Can you work these out from the drawing? Everything is in mm from the part's minimum corner. A direction names the side the tool comes from. Coordinates: 2 decimals unless noted, no trailing zeros. Order: outer loops, then holes, each group sorted by start corner. A loop starts at its lowest first (then second) coordinate and runs counter-clockwise, first axis right, second up. Notation, with made-up numbers: (-16.75, 70) -> (12.25, 70) arc R29 ccw to (12.25, 90) -> close; hole circle Ø5 at (-8.75, 30). An arc over 180 degrees is marked (long way). Answer in a Markdown table with one row per item.
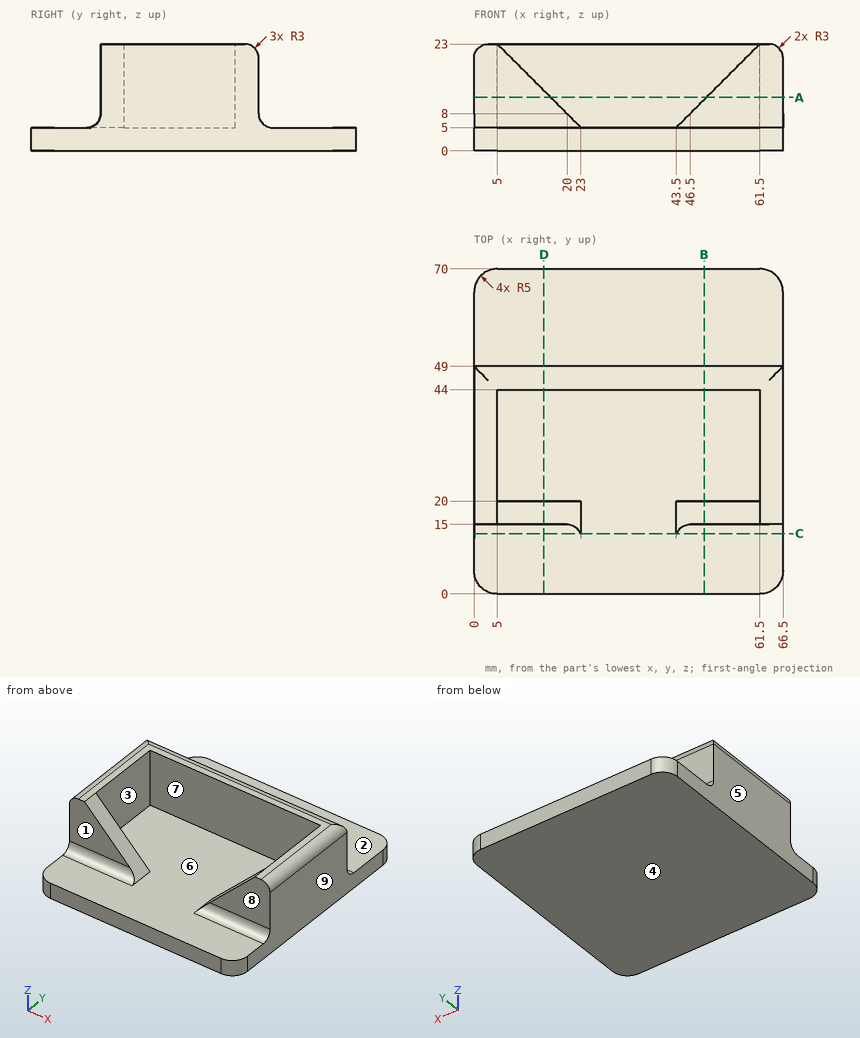
(1) Suppose I cut it at A-A (z = 11.5). Please give me the cut outline in (x, y), and give its area (4 significant figures).
Response values:
| item | result |
|---|---|
| outline | (0, 15) -> (16.5, 15) -> (16.5, 20) -> (5, 20) -> (5, 44) -> (61.5, 44) -> (61.5, 20) -> (50, 20) -> (50, 15) -> (66.5, 15) -> (66.5, 49) -> (0, 49) -> close |
| area | 737.5 mm2 |
(2) Suppose I cut it at C-C (y = 13). Please give me the cut outline in (x, z).
Response values:
| item | result |
|---|---|
| outline | (0, 0) -> (66.5, 0) -> (66.5, 5.17) -> (43.67, 5.17) -> (43.5, 5) -> (23, 5) -> (22.83, 5.17) -> (0, 5.17) -> close |
(3) I need wall thicknesses on line 1 (Y direction, x = 60, z = 19.75); line 2 (Z direction, x = 34, y = 4.5); line 3 (X direction, y = 37, z = 8.5). Which ranges of each line are inside material? Lowest first, please. Write a range as [from, to].
Response values:
| item | result |
|---|---|
| line 1 | [15, 20], [44, 49] |
| line 2 | [0, 5] |
| line 3 | [0, 5], [61.5, 66.5] |
(4) Suppose I cut it at D-D (x = 15). Please give me the cut outline in (y, z), and give its area (3 significant figures).
Response values:
| item | result |
|---|---|
| outline | (0, 0) -> (70, 0) -> (70, 5) -> (52, 5) arc R3 cw to (49, 8) -> (49, 20) arc R3 ccw to (46, 23) -> (44, 23) -> (44, 5) -> (20, 5) -> (20, 13) -> (15, 13) -> (15, 8) arc R3 cw to (12, 5) -> (0, 5) -> close |
| area | 482 mm2 |
(5) We'd pull the mould along X, two halves only. Please class the marked faces 6, 7, 8 and 9: +X half, -X half, draft (parallel to the pull), parting line (faces both ways), or undercut.
Response values:
| item | result |
|---|---|
| face 6 | undercut |
| face 7 | undercut |
| face 8 | draft |
| face 9 | +X half |
(6) Suppose I cut it at B-B (x = 49.5). Please give me the cut outline in (y, z), and give its area (3 significant figures).
Response values:
| item | result |
|---|---|
| outline | (0, 0) -> (70, 0) -> (70, 5) -> (52, 5) arc R3 cw to (49, 8) -> (49, 20) arc R3 ccw to (46, 23) -> (44, 23) -> (44, 5) -> (20, 5) -> (20, 11) -> (15, 11) -> (15, 8) arc R3 cw to (12, 5) -> (0, 5) -> close |
| area | 472 mm2 |
(7) On a 3-axis mill with a long thin cutter (end or side, diameter ignored), from which of +Z, -Z, +X, -X, +Y, -Y can I reach the whole of each face in a straight line? I mean the marked faces 1, 2, 3, 4 and 5. Say none if no direction works.
Response values:
| item | result |
|---|---|
| face 1 | +Z, +X, -X, -Y |
| face 2 | +Z, +X, -X, +Y |
| face 3 | +Z |
| face 4 | -Z, +X, -X, +Y, -Y |
| face 5 | +Z, -Z, -X, +Y, -Y |
(8) Will these pins go through, and if not, where does the flat tip stop? pin 1 Ø13 at (x, z) = (32, 16) entering from +Y; pin 2 Ø4 at (x, z) = (20.5, 14) entering from -Y; pin 3 Ø2 at (x, y) = (7, 40.5) entering from +Z.
Response values:
| item | result |
|---|---|
| pin 1 | y = 49 |
| pin 2 | y = 44 |
| pin 3 | z = 5 |
